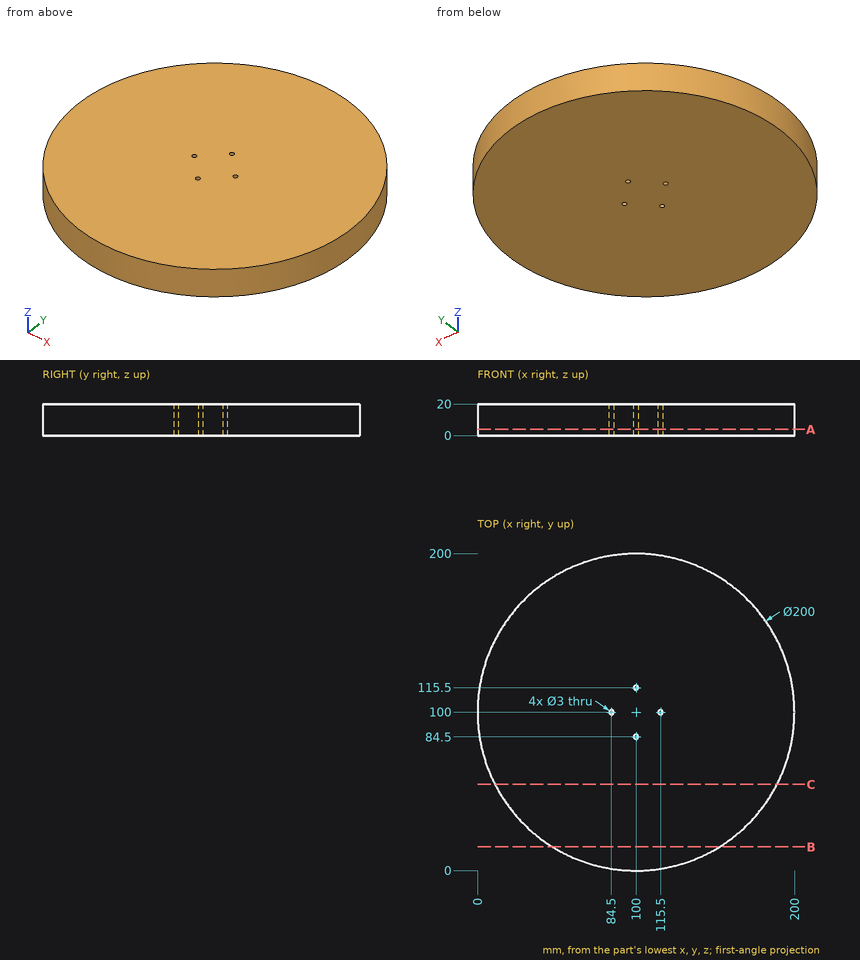
Geometry check sheet. Reference: drawing and pictorial views, mm from the part's lowest x, y, z. Give positions to 0.01 mm unless a question says otherwise; leave off trailing zeros. Order: outer loops, then holes, each group sorted by start corner. A loop starts at its lowest first (then second) coordinate and runs counter-clockwise, first axis right, second up.
1. Section check B-B, the plane y = 15. Enter the section's corners in (x, z).
2. Thickness scan on L1, parallel to Y at x = 100, z = 13.75; L2, parallel to Y at x = 102.5, z = 4.5; L3, parallel to X at y = 103, z = 8.75. Record the ranges inside material, lowest first.
3. Gauge pin test, flat ends, axial feed: pin 1 Ø4 at (x, y) = (100, 84.5) entering from +Z; pin 2 Ø8 at (x, z) = (112, 12) entering from +Y; pin 3 Ø4 at (x, z) = (108, 10.5) entering from -Y; pin 4 Ø4 at (x, z) = (50, 8) entering from -Y. Record the tip position at first contact, or that the pin passes through.
4. Section check A-A, the plane z = 4. Enter the section's corners in (x, y), and give its area (3 significant figures).
5. Section check C-C, the plane y = 54.5. Enter the section's corners in (x, z).
Values follow:
1. outline: (47.32, 0) - (152.68, 0) - (152.68, 20) - (47.32, 20) - close
2. L1: y = 0 to 83, 86 to 114, 117 to 200
2. L2: y = 0.03 to 199.97
2. L3: x = 0.05 to 199.95
3. pin 1: stops at z = 20
3. pin 2: stops at y = 199.68
3. pin 3: stops at y = 0.18
3. pin 4: stops at y = 12.27
4. outline: circle Ø200 at (100, 100); hole circle Ø3 at (84.5, 100); hole circle Ø3 at (100, 84.5); hole circle Ø3 at (100, 115.5); hole circle Ø3 at (115.5, 100)
4. area: 31,400 mm2
5. outline: (10.95, 0) - (189.05, 0) - (189.05, 20) - (10.95, 20) - close
